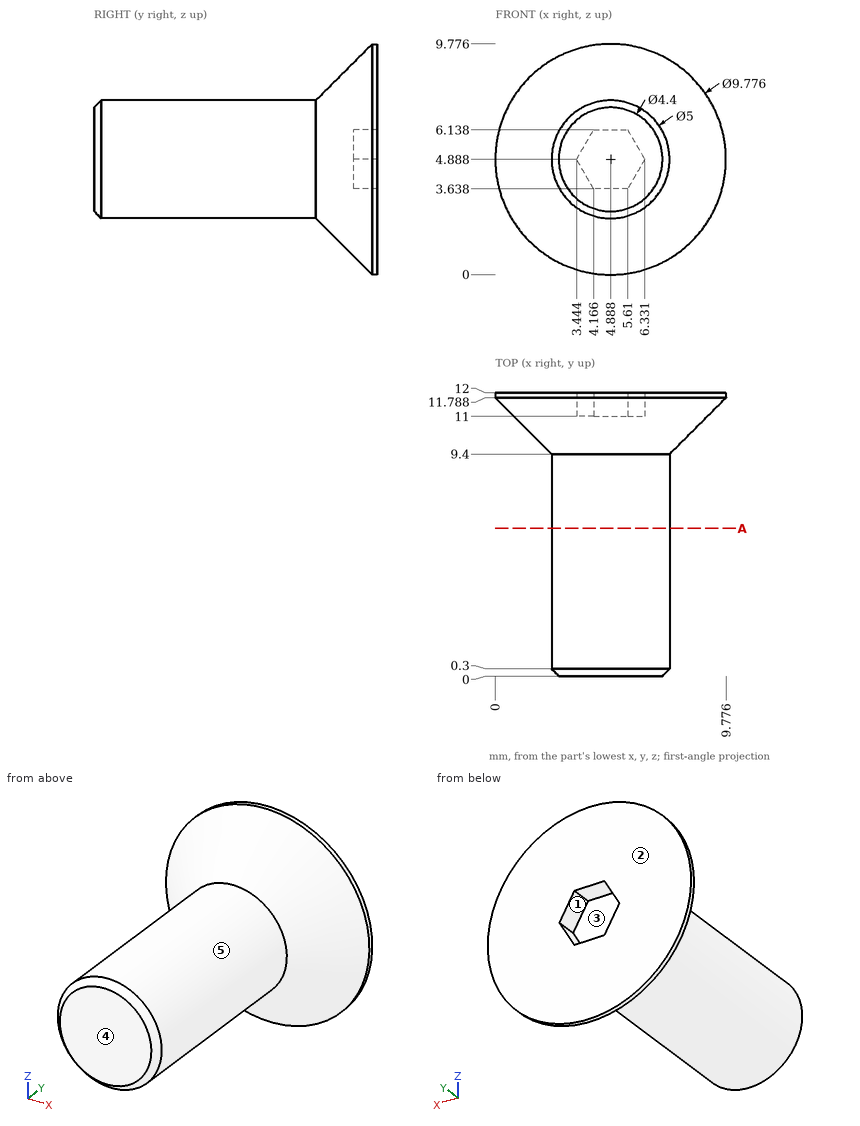
Could you check a few things on this drawing? It's one solid part, dimensions in mm from its lowest x, y, z. A direction names the side the tool comes from. Coordinates: 2 decimals unless noted, no trailing zeros. Loops run counter-clockwise (first coordinate to the right, second up) from the corner with the lowest first, then second, coordinate; pieces in that order, holes last. Notation, with made-up numbers: (23, -32.75) - (71, -32.75) arc R16 cw to (71, -2.75) - close; hole circle Ø9 at (-25.75, -35.5). An arc over 180 degrees is marked (long way). Answer as a JSON object with one key per item and string values. Group by question number.
Item 1: If I drill on L1, parallel to Y at x = 4.5, z = 6; L2, parallel to X at y = 5.25, z = 6.25 (1 decimal); L3, parallel to Z at x = 5.25, y = 8.25 (1 decimal), over which ranges is the centre line in solid material (lowest first)? Write a range as from..to.
Item 2: For pin 1 (0.8 mm diameter, centred on x = 5, z = 5, fed in from +Y); pin 2 (1.5 mm diameter, centred on y = 3, z = 5, fed in from -X); pin 3 (5 mm diameter, centred on x = 1.5, y = 1.5, fed in from -Z), each with a flat end and sliding along its axis, tell me the tip position at first contact or that it passes through.
Item 3: On a 3-axis mill with a long thin cutter (end or side, diameter ignored), from which of +Z, -Z, +X, -X, +Y, -Y can I reach the whole of each face in a straight line? I mean the marked faces 1 and 2. Say none if no direction works.
Item 4: If we section it at A-A (y = 6.25): List the corners of the cut face in (x, z) for me.
Item 5: If we mould it in two halves opening along X, with no side actions, what happens to the marked faces 3, 4 and 5? For each: released by +X, released by -X, zero draft, split by the parting line, or undercut.
Returned:
{
 "1": {"L1": "y = 0..11", "L2": "x = 2.8..7", "L3": "z = 2.4..7.4"},
 "2": {"pin 1": "stops at y = 11", "pin 2": "stops at x = 2.39", "pin 3": "stops at z = 2.55"},
 "3": {"face 1": "+Y", "face 2": "+Z, -Z, +X, -X, +Y"},
 "4": {"outline": "circle Ø5 at (4.89, 4.89)"},
 "5": {"face 3": "undercut", "face 4": "zero draft", "face 5": "split by the parting line"}
}
